The listing builds one solid part. Answer for the finished solid, in the listing's coordinates (mm). A direction names the side the tool comes from. Give positions to 0.01 mm unless a question says otherwise; leave off trailing zeros. Order: outer loops, then holes, each group sorted by start corner. A loop starts at its lowest first (then second) coordinate and runs counter-clockwise, first axis right, second up. Notation, with made-up numbers: (-21.5, 66) -> (11.5, 66) arc R16 cw to (11.5, 84) -> close; hole circle Ø10 at (33.5, -11.75). An arc over 180 degrees is marked (long way). Write item = value, one per line. Start each with the question number.
```python
from build123d import *

# Parameters (mm, degrees)
ESQUISSE1_R                  = 53.1
BOSS_EXTRU_1_DEPTH           = 25.4
ESQUISSE2_R                  = 50
BOSS_EXTRU_2_DEPTH           = 10
ESQUISSE3_R                  = 6
BOSS_EXTRU_3_DEPTH           = 34.6
R_P_TITION_CIRCULAIRE1_COUNT = 4


with BuildPart() as part:
    # Esquisse1 → Boss.-Extru.1 (new body)
    with BuildSketch(Plane.XY):
        Circle(ESQUISSE1_R)
    extrude(amount=BOSS_EXTRU_1_DEPTH)

    # Esquisse2 → Boss.-Extru.2 (add)
    with BuildSketch(Plane.XY.offset(25.4)):
        Circle(ESQUISSE2_R)
    extrude(amount=BOSS_EXTRU_2_DEPTH)

    # Esquisse3 → Boss.-Extru.3 (add)
    with BuildSketch(Plane.XY.offset(35.4)):
        with Locations((36.76305328, 17.369902519)):
            Circle(ESQUISSE3_R)
    boss_extru_3 = extrude(amount=BOSS_EXTRU_3_DEPTH)

    # R_p_tition circulaire1: Boss.-Extru.3 ×4 about axis
    r_p_tition_circulaire1_axis = Axis((0, 0, 0), (0, 0, 1))
    for i in range(1, R_P_TITION_CIRCULAIRE1_COUNT):
        add(boss_extru_3.rotate(r_p_tition_circulaire1_axis, i * 360 / R_P_TITION_CIRCULAIRE1_COUNT))


solid = part.part
```
Item 1: Which of the six approach directions +Z, -Z, +X, -X, +Y, -Y give full straight-line access (tool end or side, diameter ignored) to faces 1 (the flat face through (-37, -17, 70)), 2 (the cylindrical face through (17.63, -30.77, 52.46))?
Item 2: A cutting plane is placed at D-D, the plane z = 13. Write down the section's boundary in (x, y), plus the area to 3 significant figures.
Item 3: Consider L1, parallel to Z at x = 15.5, y = -23.5; L2, parallel to X at y = 1.5, z = 15; L3, parallel to Y at x = -37, z = 37. Determine where each line is inside the solid, lowest interval first. Write a range as from..to.
Item 4: A cutting plane is placed at C-C, the plane z = 48.5. Write down the section's boundary in (x, y), plus the area to 3 significant figures.
Item 5: Flat-ended cylindrical pins translate along their axes: pin 1 (3 mm diameter, centred on y = 0, z = 35.5, fed in from -X); pin 2 (5 mm diameter, centred on x = -31.5, y = -3.5, fed in from +Z); pin 3 (12 mm diameter, centred on y = -13.5, z = 34.5, fed in from +X). Find the tip coordinate at first contact, or state that the pin passes through.
Item 6: A cutting plane is placed at A-A, the plane y = 0. Write down the section's boundary in (x, z).
Check values:
q1.face_1 = +Z, +X, -X, +Y, -Y
q1.face_2 = +Z
q2.outline = circle Ø106.2 at (0, 0)
q2.area = 8,860 mm^2
q3.L1 = 0..35.4
q3.L2 = -53.08..53.08
q3.L3 = -23.37..-11.37
q4.outline = circle Ø12 at (-36.76, -17.37); circle Ø12 at (-17.37, 36.76); circle Ø12 at (17.37, -36.76); circle Ø12 at (36.76, 17.37)
q4.area = 452 mm^2
q5.pin_1 = -50
q5.pin_2 = 35.4
q5.pin_3 = 49.43
q6.outline = (-53.1, 0) -> (53.1, 0) -> (53.1, 25.4) -> (50, 25.4) -> (50, 35.4) -> (-50, 35.4) -> (-50, 25.4) -> (-53.1, 25.4) -> close
